from build123d import *

# Parameters (mm, degrees)
F1_DEPTH  = 25.4
F2_R      = 9.2037028664
F3_DEPTH  = 25.4
F4_W      = 16.5919382125
F4_H      = 6.8211294711
F5_DEPTH  = 25.4
F6_DEPTH  = 25.4
F8_DEPTH  = 25.4
F9_DEPTH  = 25.4
F10_R     = 4.5988805072
F11_DEPTH = 177.8


with BuildPart() as f1:
    # F0 (on Top) → F1 (new body)
    with BuildSketch(Plane.XY):
        Polygon((-29.9576614052, 52.6333078742), (-53.7394359708, 31.2481448054), (-41.9407263398, 31.2481448054), (-25.5331452936, 42.3094369471), align=None)
        Polygon((-23.8739512861, 35.303954035), (-41.9407263398, 31.2481448054), (0, 31.2481448054), align=None)
        Polygon((-25.5331452936, 42.3094369471), (-41.9407263398, 31.2481448054), (-23.8739512861, 35.303954035), align=None)
        Polygon((0, 31.2481448054), (-29.9576614052, 52.6333078742), (-25.5331452936, 42.3094369471), align=None)
        Polygon((-23.8739512861, 35.303954035), (0, 31.2481448054), (-25.5331452936, 42.3094369471), align=None)
    extrude(amount=F1_DEPTH)

    # F2 (on face) → F3 (join)
    with BuildSketch(Plane(origin=(14.7765754508, 20.6999424161, 0), x_dir=(-0.8139026255, 0.5810013049, 0), z_dir=(0.5810013049, 0.8139026255, 0))):
        with Locations((38.1454527378, 11.5221776068)):
            Circle(F2_R)
    extrude(amount=F3_DEPTH)

    # F4 (on face) → F5 (join)
    with BuildSketch(Plane(origin=(0, 0, 0), x_dir=(1, 0, 0), z_dir=(0, 0, -1))):
        with Locations((-28.4828236327, -38.5301616043)):
            Rectangle(F4_W, F4_H)
    extrude(amount=F5_DEPTH)

    # F6 (add): a face of the model
    f6_faces = [f1.faces().sort_by_distance(p)[0] for p in [
        (-28.4828236327, 38.5301616043, -25.4),
    ]]
    extrude(f6_faces, amount=F6_DEPTH)

    # F7 (on face) → F8 (join)
    with BuildSketch(Plane(origin=(29.5340085947, 41.3730691028, 0), x_dir=(-0.8139026255, 0.5810013049, 0), z_dir=(0.5810013049, 0.8139026255, 0))):
        Polygon((45.5019623041, 7.2748948284), (45.5019623041, 15.7694603852), (38.1454527378, 20.0167431636), (30.7889431715, 15.7694603852), (30.7889431715, 7.2748948284), (38.1454527378, 3.02761205), align=None)
    extrude(amount=F8_DEPTH)

    # F9 (add): a face of the model
    f9_faces = [f1.faces().sort_by_distance(p)[0] for p in [
        (13.244757606, 84.2087536053, 11.5221776068),
    ]]
    extrude(f9_faces, amount=F9_DEPTH)

    # F10 (on face) → F11 (join)
    with BuildSketch(Plane(origin=(59.0488748825, 82.7193224761, 0), x_dir=(-0.8139026255, 0.5810013049, 0), z_dir=(0.5810013049, 0.8139026255, 0))):
        with Locations((38.1127148867, 11.3378223032)):
            Circle(F10_R)
    extrude(amount=F11_DEPTH)


solid = f1.part
Could you check a few things on this model? Use its own coordinates, in mm. A direction names the side the tool comes from. Give positions to 0.01 mm unless a question says otherwise; leave off trailing zeros. Order: outer loops, then holes, each group sorted by start corner. A loop starts at its lowest first (then second) coordinate and runs counter-clockwise, first axis right, second up. Notation, with made-up numbers: M 76,24 L 88,24 A25 ccw 88,38 Z; hole C 4,-29.75 d1. An arc over 180 degrees is marked long. One line per question, with ' | ' between items.
1. I want a section at A-A (x = 16). List the corners of the cut face in (y, z) for me, and give its area (3 significant figures).
Results:
outline: M 75.41,7.27 L 88.07,3.03 L 100.73,7.27 L 100.73,15.77 L 88.07,20.02 L 75.41,15.77 Z | area: 323 mm²
2. If I drill on line 1 (X direction, y = 144.5, z = 11); line 2 (X direction, y = 116.5, z = 8.5); line 3 (Y direction, x = 50, z = 14), over which ranges is the centre line in solid material (lowest first)?
Results:
line 1: 50.69 to 61.96 | line 2: 31.89 to 40.78 | line 3: 129.19 to 142.1
3. For faces 5 (the face through (-36.779, 39, -25)), 6 (the face through (-4.25, 65.49, 18.38)), 7 (the face through (131.38, 249.54, 11.4)), 8 (the face through (-29, 38, -50.8)), 9 (the face through (-20.187, 39, -25)), which set-ups out of +Z, -Z, +X, -X, +Y, -Y let a thin tool reach every point of the face, with its end or its side?
Results:
face 5: -Z, -X, +Y, -Y | face 6: none | face 7: +Z, -Z, +X, +Y | face 8: -Z, +X, -X, +Y, -Y | face 9: -Z, +X, +Y, -Y
4. We'd pull the mould along X, two halves only. Please class faces 1 (the face through (-41.68, 42.09, 12.52)), 2 (the face through (19.03, 79.65, 11.58)), 3 (the face through (30.75, 102.92, 7.87)), 4 (the face through (-29, 35.12, -25)): +X half, -X half, draft (parallel to the pull), parting line (faces both ways), or undercut.
Results:
face 1: -X half | face 2: +X half | face 3: undercut | face 4: draft
5. I'm going to push flat-ended pins straight in: pin 1 (5 mm diameter, centred on x = -32.5, z = -34.5, fed in from -Y); pin 2 (7.5 mm diameter, centred on y = 39.5, z = -28, fed in from -X); pin 3 (1.5 mm diameter, centred on x = 59, y = 140.5, fed in from -Z). Where does each tip first touch, or does it pass through?
Results:
pin 1: y = 35.12 | pin 2: x = -36.78 | pin 3: z = 8.68
6. I want a section at B-B (z = -6). List the corners of the cut face in (x, y) for me, and give its area (3 significant figures).
Results:
outline: M -36.78,35.12 L -20.19,35.12 L -20.19,41.94 L -36.78,41.94 Z | area: 113 mm²
